from build123d import *

# Parameters (mm, degrees)
SKETCH2_W               = 165.1
SKETCH2_H               = 177.8
BOSS_EXTRUDE1_DEPTH     = 13.97
FILLET1_R               = 16.51
SKETCH3_R               = 1.905
CUT_EXTRUDE1_DEPTH      = 123.118276273
BOSS_EXTRUDE2_DEPTH     = 4.445
CUT_EXTRUDE3_DEPTH      = 123.118276273
CUT_EXTRUDE3_DEPTH_BACK = 123.118276273
SKETCH4_R               = 13.335
SKETCH9_R               = 69.85
CUT_EXTRUDE4_DEPTH      = 2.921
CUT_EXTRUDE5_DEPTH      = 17.145


with BuildPart() as part:
    # Sketch2 → Boss-Extrude1 (new body)
    with BuildSketch(Plane(origin=(0, 0, 0), x_dir=(1, 0, 0), z_dir=(0, 1, 0))):
        Rectangle(SKETCH2_W, SKETCH2_H)
    extrude(amount=BOSS_EXTRUDE1_DEPTH)

    # Fillet1
    fillet1_edges = [part.edges().sort_by_distance(p)[0] for p in [
        (82.55, 6.985, 88.9),
        (-82.55, 6.985, 88.9),
        (-82.55, 6.985, -88.9),
        (82.55, 6.985, -88.9),
    ]]
    fillet(fillet1_edges, radius=FILLET1_R)

    # Sketch3 → Cut-Extrude1 (cut, through all)
    with BuildSketch(Plane.XZ):
        with Locations(Location((-63.5, 71.12, 0), (0, 0, 270))):
            Circle(SKETCH3_R)
        with Locations(Location((63.5, 71.12, 0), (0, 0, 270))):
            Circle(SKETCH3_R)
        with Locations(Location((-63.5, -71.12, 0), (0, 0, 270))):
            Circle(SKETCH3_R)
        with Locations(Location((63.5, -71.12, 0), (0, 0, 270))):
            Circle(SKETCH3_R)
    extrude(amount=-CUT_EXTRUDE1_DEPTH, mode=Mode.SUBTRACT)

    # Sketch5 → Boss-Extrude2 (add)
    with BuildSketch(Plane.XZ):
        with BuildLine():
            Line((-49.252427351, 49.53), (49.252427351, 49.53))
            ThreePointArc((49.252427351, 49.53), (0, -69.85), (-49.252427351, 49.53))
        make_face()
    extrude(amount=BOSS_EXTRUDE2_DEPTH)

    # Sketch4 → Cut-Extrude3 (cut, two sides: drawn at the far end of the back side and taken through both)
    with BuildSketch(Plane.XZ.offset(-CUT_EXTRUDE3_DEPTH_BACK)):
        with Locations(Location((0, 0, 0), (0, 0, 270))):
            Circle(SKETCH4_R)
    extrude(amount=CUT_EXTRUDE3_DEPTH + CUT_EXTRUDE3_DEPTH_BACK, mode=Mode.SUBTRACT)

    # Sketch9 → Cut-Extrude4 (cut)
    with BuildSketch(Plane(origin=(0, 13.97, 0), x_dir=(1, 0, 0), z_dir=(0, 1, 0))):
        with Locations(Location((0, 0, 0), (0, 0, 270))):
            Circle(SKETCH9_R)
    extrude(amount=-CUT_EXTRUDE4_DEPTH, mode=Mode.SUBTRACT)

    # Sketch15 → Cut-Extrude5 (cut, symmetric)
    with BuildSketch(Plane(origin=(0, 0, 0), x_dir=(0, 0, -1), z_dir=(1, 0, 0))):
        Polygon((-51.562, 11.049), (-51.562, -5.08), (-29.972, 11.049), align=None)
    extrude(amount=CUT_EXTRUDE5_DEPTH, both=True, mode=Mode.SUBTRACT)


solid = part.part
Geometry check sheet. Reference: the model listing, model coordinates, mm. A direction names the side the tool comes from. Give positions to 0.01 mm unless a question says otherwise; leave off trailing zeros. Loops run counter-clockwise (first coordinate to the right, second up) from the corner with the lowest first, then second, coordinate; pieces in that order, holes last. Notation, with made-up numbers: (19, 23) -> (34, 23) arc R13 cw to (34, 28) -> close; hole circle Ø11 at (14, 6.25). An arc over 180 degrees is marked (long way). Answer in a Markdown table with one row per item. Add a question column.
1) Material ranges on probe 1 along X at (y, z) = (3.75, 71.12) (3 decimals); probe 2 along Y at (x, z) = (-11, -35) (3 decimals); probe 3 along Y at (x, z) = (-67, 65.5), recorded low to high. Write a range as from..to.
2) Cross-section at A-A on x = 0. Record the boundary of the cut face in (y, z) (3 decimals).
3) Cross-section at C-C on y = 3. Record the boundary of the cut face in (x, z) (3 decimals).
4) Draft check along X on faces 1 (the face through (0.24, 3.64, 39.89)), 2 (the face through (82.55, 7, 1)), 3 (the face through (-82.55, 7, 1)). Enter one of: pulls with the +X half, pulls with the -X half, needs draft (parallel to the pull), parting line crosses it, or undercut.
5) Cross-section at B-B on z = -9. Record the boundary of the cut face in (x, y) (3 decimals).
6) Gauge pin test, flat ends, axial feed: P1, Ø8, axis at x = 55.5, z = -55, coming from the -Y side; P2, Ø6, axis at x = 63.5, z = -71.12, coming from the +Y side. Record the tip position at first contact, or that the pin passes through.
7) Cross-section at D-D on z = 47.5. Record the boundary of the cut face in (x, y) (3 decimals).
8) Set-up check for faces 4 (the face through (0, 6, 51.562)), 5 (the face through (17.145, 7, 43)), 6 (the face through (-1, -4, 49.53)): record each of +Z, -Z, +X, -X, +Y, -Y from which the full face is reachable in a straight line by a thin tool's end or side.
Outcome:
| question | item | result |
|---|---|---|
| 1 | probe 1 | x = -82.55..-65.405, -61.595..61.595, 65.405..82.55 |
| 1 | probe 2 | y = -4.445..11.049 |
| 1 | probe 3 | y = 0..13.97 |
| 2 | outline | (-4.445, -69.85) -> (0, -69.85) -> (0, -88.9) -> (13.97, -88.9) -> (13.97, -69.85) -> (11.049, -69.85) -> (11.049, -13.335) -> (-4.445, -13.335) -> close; (-4.445, 13.335) -> (11.049, 13.335) -> (11.049, 29.972) -> (-3.562, 49.53) -> (-4.445, 49.53) -> close; (0, 51.562) -> (11.049, 51.562) -> (11.049, 69.85) -> (13.97, 69.85) -> (13.97, 88.9) -> (0, 88.9) -> close |
| 3 | outline | (-82.55, -72.39) arc R16.51 ccw to (-66.04, -88.9) -> (66.04, -88.9) arc R16.51 ccw to (82.55, -72.39) -> (82.55, 72.39) arc R16.51 ccw to (66.04, 88.9) -> (-66.04, 88.9) arc R16.51 ccw to (-82.55, 72.39) -> close; hole circle Ø3.81 at (-63.5, -71.12); hole circle Ø3.81 at (-63.5, 71.12); hole (-17.145, 40.746) -> (17.145, 40.746) -> (17.145, 51.562) -> (-17.145, 51.562) -> close; hole circle Ø26.67 at (0, 0); hole circle Ø3.81 at (63.5, -71.12); hole circle Ø3.81 at (63.5, 71.12) |
| 4 | face 1 | undercut |
| 4 | face 2 | pulls with the +X half |
| 4 | face 3 | pulls with the -X half |
| 5 | outline | (-82.55, 0) -> (-69.268, 0) -> (-69.268, -4.445) -> (-9.84, -4.445) -> (-9.84, 11.049) -> (-69.268, 11.049) -> (-69.268, 13.97) -> (-82.55, 13.97) -> close; (9.84, -4.445) -> (69.268, -4.445) -> (69.268, 0) -> (82.55, 0) -> (82.55, 13.97) -> (69.268, 13.97) -> (69.268, 11.049) -> (9.84, 11.049) -> close |
| 6 | P1 | stops at y = 0 |
| 6 | P2 | stops at y = 13.97 |
| 7 | outline | (-82.55, 0) -> (-51.213, 0) -> (-51.213, -4.445) -> (51.213, -4.445) -> (51.213, 0) -> (82.55, 0) -> (82.55, 13.97) -> (51.213, 13.97) -> (51.213, 11.049) -> (17.145, 11.049) -> (17.145, -2.045) -> (-17.145, -2.045) -> (-17.145, 11.049) -> (-51.213, 11.049) -> (-51.213, 13.97) -> (-82.55, 13.97) -> close |
| 8 | face 4 | +Y, -Y |
| 8 | face 5 | +Y |
| 8 | face 6 | +Z, +X, -X, -Y |
